Could you check a few things on this drawing? It's one solid part, dimensions in mm from its lowest x, y, z. A direction names the side the tool comes from. Coordinates: 2 decimals unless noted, no trailing zeros. Write each loop counter-clockwise with the first axis right and the second up, starting at its lowest first coordinate (ties: lowest second). Pieces come first, ordered by that corner, then holes.
Item 1: Please list where these lines run through material, in increasing order: line 1 (Y direction, x = 9.5, z = 2.75); line 2 (X direction, y = 10.75, z = 10.75); line 3 (X direction, y = 8.25, z = 5).
Item 2: I'm going to push flat-ended pins straight in: P1, Ø1, axis at x = 13, z = 6, coming from the +Y side (1 decimal); P2, Ø10, axis at x = 13.5, y = 3.5, coming from the -Z side. Where does each tip first touch, or does it pass through?
Item 3: For the marked faces 5 and 6, which set-ups out of +Z, -Z, +X, -X, +Y, -Y let a thin tool reach every point of the face, with its end or its side?
Item 4: I want a section at B-B (y = 8.5). Please give me the cut outline in (x, z), and give its area (3 significant figures).
Item 5: If we mould it in two halves opening along X, with no side actions, what happens to the marked faces 1, 2, 3 and 4? For each: pulls with the +X half, pulls with the -X half, needs draft (parallel to the pull), parting line crosses it, or undercut.
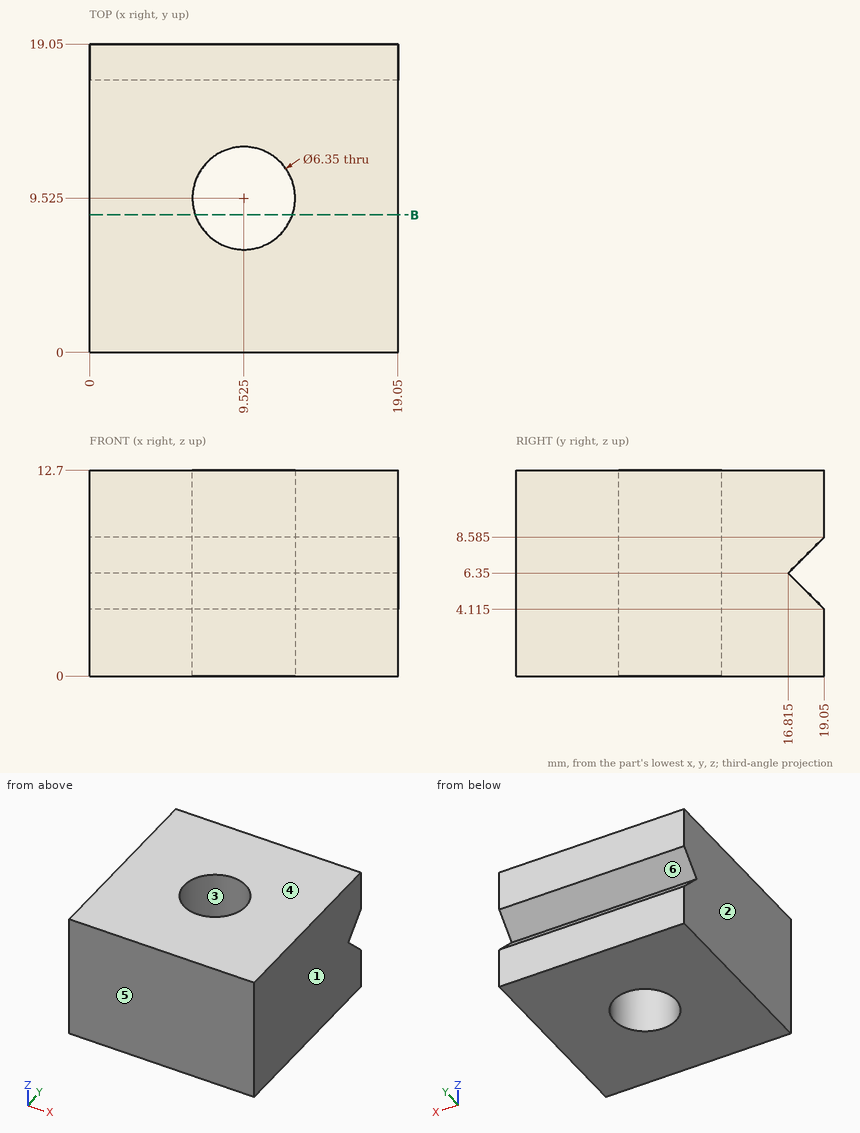
Answer:
1. line 1: y = 0 to 6.35, 12.7 to 19.05
1. line 2: x = 0 to 6.6, 12.45 to 19.05
1. line 3: x = 0 to 6.62, 12.43 to 19.05
2. P1: stops at y = 17.7
2. P2: stops at z = 0
3. face 5: +Z, -Z, +X, -X, -Y
3. face 6: +X, -X, +Y
4. outline: (0, 0) - (6.52, 0) - (6.52, 12.7) - (0, 12.7) - close; (12.53, 0) - (19.05, 0) - (19.05, 12.7) - (12.53, 12.7) - close
4. area: 166 mm2
5. face 1: pulls with the +X half
5. face 2: pulls with the -X half
5. face 3: undercut
5. face 4: needs draft
